For this review, use the dimensioned drawing (mm, ordinates from the lowest corner) and the shaded views. Round coordinates to 2 decimals unless told otherwise and drop trailing zeros. Write each loop counter-clockwise with the first axis right and the second up, starting at its lowest first coordinate (ties: lowest second). Pieces come first, ordered by that corner, then holes. Notation, with made-up numbers: M 11.5,56.25 L 37.5,56.25 A18 cw 37.5,68.25 Z; hole C 87,79.5 d4. An arc over 180 degrees is marked long. Use one line per item in the form item = value. Start each with the question number.
Item 1: Add section A-A (x = 24.39). State the section outline as (y, z) points (3 decimals).
Item 2: For line 1 (X direction, y = 0.8, z = 2.5); line 2 (X direction, y = 1.3, z = 30) (3 decimals); line 3 (Z direction, x = 9.5, y = 1.55) (3 decimals), list the stretches that pass through material, from the lowest coordinate up. Write a range as [from, to].
Item 3: Add section C-C (x = 28.5). State the section outline as (y, z) points, and give its area (3 significant figures).
Item 4: For P1, Ø0.8, axis at y = 2.5, z = 31, coming from the -X side (3 decimals); P2, Ø2.5, axis at x = 28.5, z = 2.5, coming from the +Y side; P3, Ø1.9, axis at x = 2.5, z = 2.5, coming from the +Y side; P4, Ø0.5, axis at x = 16.5, y = 1.5, coming from the +Z side (3 decimals), all flat-tipped, find the tip position at first contact; note any pin that passes through.
Item 5: Add section B-B (z = 33). State the section outline as (x, y) points (3 decimals), and give its area (3 significant figures).
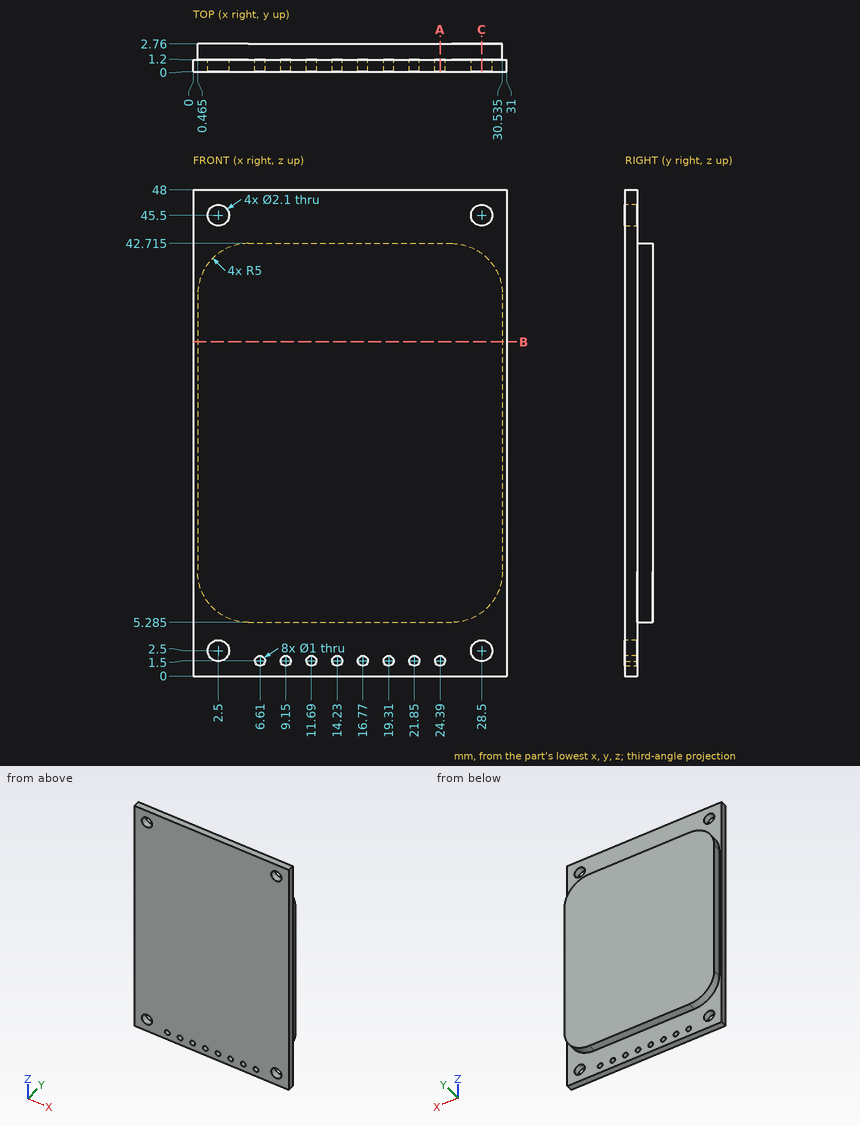
Calculated:
q1.outline = M 0,0 L 1.2,0 L 1.2,1 L 0,1 Z; M 0,2 L 1.2,2 L 1.2,5.285 L 2.76,5.285 L 2.76,42.715 L 1.2,42.715 L 1.2,48 L 0,48 Z
q2.line_1 = [0, 1.45], [3.55, 27.45], [29.55, 31]
q2.line_2 = [0.465, 30.535]
q2.line_3 = [5.285, 42.715]
q3.outline = M 0,0 L 1.2,0 L 1.2,1.45 L 0,1.45 Z; M 0,3.55 L 1.2,3.55 L 1.2,6.26 L 2.76,6.26 L 2.76,41.74 L 1.2,41.74 L 1.2,44.45 L 0,44.45 Z; M 0,46.55 L 1.2,46.55 L 1.2,48 L 0,48 Z
q3.area = 108 mm^2
q4.P1 = 0.465
q4.P2 = 1.2
q4.P3 = through
q4.P4 = 42.715
q5.outline = M 0,0 L 31,0 L 31,1.2 L 30.535,1.2 L 30.535,2.76 L 0.465,2.76 L 0.465,1.2 L 0,1.2 Z
q5.area = 84.1 mm^2
